Read the model definition and answer for the solid it produces. Units are mm, in the model's axes. Coordinates: 2 decimals unless noted, no trailing zeros. Order: outer loops, then holes, each group sorted by start corner. A loop starts at its lowest first (then second) coordinate and runs counter-clockwise, first axis right, second up. Notation, with made-up numbers: (-2, 89) -> (54, 89) arc R9 cw to (54, 98) -> close; hole circle Ø6 at (15.25, 65). An arc over 180 degrees is marked (long way). Answer as a JSON object with one key per item and string values. Group by question number.
1) Section B-B on z = -4.75 is taken. Determine the outline of the cut face in (x, y) (3 decimals).
2) Given pin 1 (2 mm diameter, centred on y = 5, z = -4, fed in from +X); pin 2 (4 mm diameter, centred on x = 3.5, y = 7, fed in from -Z); pin 3 (4 mm diameter, centred on x = 3.35, y = 4, fed in from -Z), each flat-ended and moving along its own axis, determine where each tip first touches the part or whether it passes through.
3) Section D-D on x = 6.75 is taken. Determine the outline of the cut face in (y, z), and give its area (3 significant figures).
4) Section A-A on x = 2 is taken. Determine the outline of the cut face in (y, z), and give its area (3 significant figures).
5) Consider L1, parallel to Y at x = 3.35, z = -0.9; L2, parallel to Z at x = 3.5, y = 2; L3, parallel to Y at x = 2.75, z = -5.25. Determine where each line is inside the solid, lowest interval first.
6) Determine the mould class of faces 1 (the flat face through (3, 2, -2.845)), 2 (the flat face through (4, 2, 0)), 3 (the cylindrical face through (0.42, 2.78, -4.62)), 4 (the cylindrical face through (13.2, 3.94, -3.99)) for opening direction X: released by +X, released by -X, zero draft, split by the parting line, or undercut.
7) Section C-C on z = -2.5 is taken. Determine the outline of the cut face in (x, y).
from build123d import *

# Parameters (mm, degrees)
BOSS_EXTRUDE1_DEPTH                            = 8
CBORE_FOR_6_SOCKET_HEAD_CAP_SCREW1_D           = 3.6576
CBORE_FOR_6_SOCKET_HEAD_CAP_SCREW1_CBORE_D     = 6.35
CBORE_FOR_6_SOCKET_HEAD_CAP_SCREW1_CBORE_DEPTH = 3.5052
CUT_EXTRUDE1_DEPTH                             = 9.0000001


with BuildPart() as part:
    # Sketch1 → Boss-Extrude1 (new body)
    with BuildSketch(Plane(origin=(0, 0, 0), x_dir=(1, 0, 0), z_dir=(0, 1, 0))):
        with BuildLine():
            Line((0, 0), (0, 6.35))
            ThreePointArc((0, 6.35), (10.998522628, 4.727972806), (21.060567419, 0))
            Line((21.060567419, 0), (0, 0))
        make_face()
    extrude(amount=BOSS_EXTRUDE1_DEPTH)

    # CBORE for #6 Socket Head Cap Screw1 (through all)
    with Locations(Plane(origin=(0, 0, -6.35), x_dir=(-1, 0, 0), z_dir=(0, 0, -1))):
        with Locations((-3.35, 4)):
            CounterBoreHole(CBORE_FOR_6_SOCKET_HEAD_CAP_SCREW1_D / 2, CBORE_FOR_6_SOCKET_HEAD_CAP_SCREW1_CBORE_D / 2, CBORE_FOR_6_SOCKET_HEAD_CAP_SCREW1_CBORE_DEPTH)

    # Sketch8 → Cut-Extrude1 (cut, through all)
    with BuildSketch(Plane.XZ):
        with BuildLine():
            Line((7.202330007, 0), (7, 0))
            Line((7, 0), (7, 1.396675329))
            Line((7, 1.396675329), (19, 1.396675329))
            Line((19, 1.396675329), (19, 0))
            ThreePointArc((19, 0), (18.911811713, -0.028662347), (18.85732587, -0.103695652))
            ThreePointArc((18.85732587, -0.103695652), (18.66092377, -0.451002442), (18.34436725, -0.693876404))
            ThreePointArc((18.34436725, -0.693876404), (18.101165003, -0.75), (17.857962756, -0.693876404))
            ThreePointArc((17.857962756, -0.693876404), (17.541406237, -0.451002442), (17.345004137, -0.103695652))
            ThreePointArc((17.345004137, -0.103695652), (17.290518293, -0.028662347), (17.202330007, 0))
            Line((17.202330007, 0), (17, 0))
            ThreePointArc((17, 0), (16.911811713, -0.028662347), (16.85732587, -0.103695652))
            ThreePointArc((16.85732587, -0.103695652), (16.66092377, -0.451002442), (16.34436725, -0.693876404))
            ThreePointArc((16.34436725, -0.693876404), (16.101165003, -0.75), (15.857962756, -0.693876404))
            ThreePointArc((15.857962756, -0.693876404), (15.541406237, -0.451002442), (15.345004137, -0.103695652))
            ThreePointArc((15.345004137, -0.103695652), (15.290518293, -0.028662347), (15.202330007, 0))
            Line((15.202330007, 0), (15, 0))
            ThreePointArc((15, 0), (14.911811713, -0.028662347), (14.85732587, -0.103695652))
            ThreePointArc((14.85732587, -0.103695652), (14.66092377, -0.451002442), (14.34436725, -0.693876404))
            ThreePointArc((14.34436725, -0.693876404), (14.101165003, -0.75), (13.857962756, -0.693876404))
            ThreePointArc((13.857962756, -0.693876404), (13.541406237, -0.451002442), (13.345004137, -0.103695652))
            ThreePointArc((13.345004137, -0.103695652), (13.290518293, -0.028662347), (13.202330007, 0))
            Line((13.202330007, 0), (13, 0))
            ThreePointArc((13, 0), (12.911811713, -0.028662347), (12.85732587, -0.103695652))
            ThreePointArc((12.85732587, -0.103695652), (12.66092377, -0.451002442), (12.34436725, -0.693876404))
            ThreePointArc((12.34436725, -0.693876404), (12.101165003, -0.75), (11.857962756, -0.693876404))
            ThreePointArc((11.857962756, -0.693876404), (11.541406237, -0.451002442), (11.345004137, -0.103695652))
            ThreePointArc((11.345004137, -0.103695652), (11.290518293, -0.028662347), (11.202330007, 0))
            Line((11.202330007, 0), (11, 0))
            ThreePointArc((11, 0), (10.911811713, -0.028662347), (10.85732587, -0.103695652))
            ThreePointArc((10.85732587, -0.103695652), (10.66092377, -0.451002442), (10.34436725, -0.693876404))
            ThreePointArc((10.34436725, -0.693876404), (10.101165003, -0.75), (9.857962756, -0.693876404))
            ThreePointArc((9.857962756, -0.693876404), (9.541406237, -0.451002442), (9.345004137, -0.103695652))
            ThreePointArc((9.345004137, -0.103695652), (9.290518293, -0.028662347), (9.202330007, 0))
            Line((9.202330007, 0), (9, 0))
            ThreePointArc((9, 0), (8.911811713, -0.028662347), (8.85732587, -0.103695652))
            ThreePointArc((8.85732587, -0.103695652), (8.66092377, -0.451002442), (8.34436725, -0.693876404))
            ThreePointArc((8.34436725, -0.693876404), (8.101165003, -0.75), (7.857962756, -0.693876404))
            ThreePointArc((7.857962756, -0.693876404), (7.541406237, -0.451002442), (7.345004137, -0.103695652))
            ThreePointArc((7.345004137, -0.103695652), (7.290518293, -0.028662347), (7.202330007, 0))
        make_face()
    extrude(amount=-CUT_EXTRUDE1_DEPTH, mode=Mode.SUBTRACT)


solid = part.part
Worked answers:
{
 "1": {"outline": "(0, 0) -> (10.925, 0) -> (10.925, 8) -> (0, 8) -> close; hole circle Ø6.35 at (3.35, 4)"},
 "2": {"pin 1": "stops at x = 15.62", "pin 2": "stops at z = -6.32", "pin 3": "stops at z = -2.84"},
 "3": {"outline": "(0, -5.75) -> (8, -5.75) -> (8, 0) -> (0, 0) -> close", "area": "46.0 mm²"},
 "4": {"outline": "(0, -6.3) -> (1.13, -6.3) -> (1.13, -2.84) -> (2.77, -2.84) -> (2.77, 0) -> (0, 0) -> close; (5.23, -2.84) -> (6.87, -2.84) -> (6.87, -6.3) -> (8, -6.3) -> (8, 0) -> (5.23, 0) -> close", "area": "23.5 mm²"},
 "5": {"L1": "y = 0 to 2.17, 5.83 to 8", "L2": "z = -2.84 to 0", "L3": "y = 0 to 0.88, 7.12 to 8"},
 "6": {"face 1": "undercut", "face 2": "zero draft", "face 3": "undercut", "face 4": "released by +X"},
 "7": {"outline": "(0, 0) -> (16.69, 0) -> (16.69, 8) -> (0, 8) -> close; hole circle Ø3.66 at (3.35, 4)"}
}
